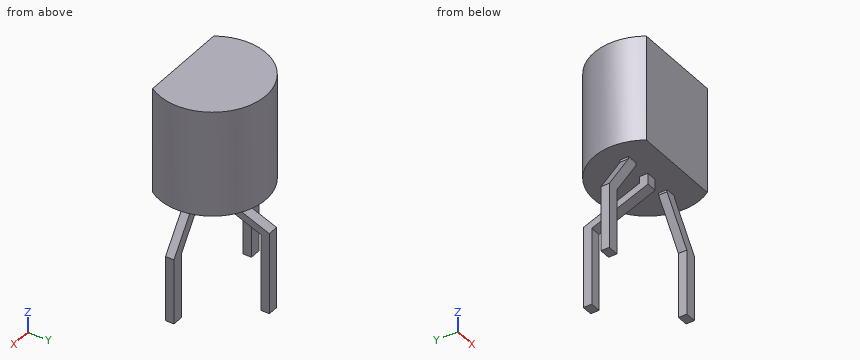
from build123d import *

# Parameters (mm, degrees)
PAD001_DEPTH = 0.19
PAD_DEPTH    = 4.8
PAD002_DEPTH = 0.24


with BuildPart() as pad001:
    # Sketch001 → Pad001 (new body, symmetric)
    with BuildSketch(Plane.XZ):
        Polygon((0.25, -2.46), (-0.25, -2.46), (-0.25, 0.5), (1.02, 2.4), (1.02, 3.04), (1.52, 3.04), (1.52, 2.4), (0.25, 0.5), align=None)
        Polygon((3.56, 3.04), (4.06, 3.04), (4.06, 2.4), (5.37, 0.5), (5.37, -2.46), (4.87, -2.46), (4.87, 0.5), (3.56, 2.4), align=None)
    extrude(amount=PAD001_DEPTH, both=True)


with BuildPart() as pad:
    # Sketch → Pad (new body)
    with BuildSketch(Plane.XY.offset(2.5)):
        with BuildLine():
            Line((0.524231, -1.33), (4.555769, -1.33))
            ThreePointArc((4.555769, -1.33), (2.54, 2.415), (0.524231, -1.33))
        make_face()
    extrude(amount=PAD_DEPTH)


with BuildPart() as to_92_wide:
    # Sketch002 → Pad002 (new body, symmetric)
    with BuildSketch(Plane.YZ.offset(2.54)):
        Polygon((-0.19, 2.5), (0.19, 2.5), (0.19, 2.2), (2.73, 1.2), (2.73, -2.5), (2.35, -2.5), (2.35, 1), (-0.19, 2), align=None)
    extrude(amount=PAD002_DEPTH, both=True)

    add(pad001.part)
    add(pad.part)


solid = to_92_wide.part
Work out the finished part from the listing and answer in its coordinate system (mm). Give positions to 0.01 mm unless a question says otherwise; leave off trailing zeros. Loops run counter-clockwise (first coordinate to the right, second up) from the corner with the lowest first, then second, coordinate; pieces in that order, holes last. Notation, with made-up numbers: (14.25, 89.25) -> (25.25, 89.25) arc R22 cw to (25.25, 98.25) -> close; hole circle Ø10 at (46, 30.5). An arc over 180 degrees is marked (long way). Use a Markdown table: item, result. Add a question column.
1. Flat-ended cylindrical pins translate along their axes: pin 1 Ø0.5 at (x, z) = (4.5, 0.5) entering from +Y; pin 2 Ø1 at (y, z) = (2, 1.5) entering from -X; pin 3 Ø1 at (x, y) = (3, 0) entering from -Z; pin 4 Ø1.9 at (x, z) = (0.5, 1) entering from +Y. Find the tip coordinate at first contact, or state that the pin passes through.
2. Section A-A on z = 0.25 is taken. Determine the outline of the cut face in (x, y), and give its area (3 significant figures).
3. Find the intervals of material crossed by probe 1 along X at (y, z) = (1.4, 1.5); probe 2 along Z at (x, y) = (3.3, -0.4); probe 3 along Y at (x, z) = (1.55, 3.5), in increasing order.
4. Section C-C on x = 0.65 is taken. Determine the outline of the cut face in (y, z).
5. Section D-D on x = 2.54 is taken. Determine the outline of the cut face in (y, z) (3 decimals).
6. Section B-B on y = 1.95 is taken. Determine the outline of the cut face in (x, z), and give its area (3 significant figures).
Results below:
| question | item | result |
|---|---|---|
| 1 | pin 1 | passes through |
| 1 | pin 2 | stops at x = 2.3 |
| 1 | pin 3 | stops at z = 1.75 |
| 1 | pin 4 | stops at y = 0.19 |
| 2 | outline | (-0.25, -0.19) -> (0.25, -0.19) -> (0.25, 0.19) -> (-0.25, 0.19) -> close; (2.3, 2.35) -> (2.78, 2.35) -> (2.78, 2.73) -> (2.3, 2.73) -> close; (4.87, -0.19) -> (5.37, -0.19) -> (5.37, 0.19) -> (4.87, 0.19) -> close |
| 2 | area | 0.562 mm^2 |
| 3 | probe 1 | x = 2.3 to 2.78 |
| 3 | probe 2 | z = 2.5 to 7.3 |
| 3 | probe 3 | y = -1.33 to 2.2 |
| 4 | outline | (-1.33, 2.5) -> (1.5, 2.5) -> (1.5, 7.3) -> (-1.33, 7.3) -> close; (-0.19, 1.1) -> (0.19, 1.1) -> (0.19, 1.85) -> (-0.19, 1.85) -> close |
| 5 | outline | (-1.33, 2.5) -> (-0.19, 2.5) -> (-0.19, 2) -> (2.35, 1) -> (2.35, -2.5) -> (2.73, -2.5) -> (2.73, 1.2) -> (0.19, 2.2) -> (0.19, 2.5) -> (2.415, 2.5) -> (2.415, 7.3) -> (-1.33, 7.3) -> close |
| 6 | outline | (1.12, 2.5) -> (3.96, 2.5) -> (3.96, 7.3) -> (1.12, 7.3) -> close; (2.3, 1.16) -> (2.78, 1.16) -> (2.78, 1.51) -> (2.3, 1.51) -> close |
| 6 | area | 13.8 mm^2 |
